```python
from build123d import *

# Parameters (mm, degrees)
F0_W     = 9
F0_H     = 6.4
F0_H_2   = 1.8
F1_DEPTH = 10
F3_DEPTH = 68.4572498646


with BuildPart() as f1:
    # F0 (on Top) → F1 (new body)
    with BuildSketch(Plane.XY):
        with BuildLine():
            Line((-23, -13.2790561914), (-23, -19.4471))
            Line((-23, -19.4471), (-23, -19.4592028655))
            ThreePointArc((-23, -19.4592028655), (-15.9535433508, -25.5567022661), (-7.3808786516, -29.2093))
            Line((-7.3808786516, -29.2093), (0, -29.2093))
            Line((0, -29.2093), (0, 0))
            Line((0, 0), (-11.5, -19.918584287))
            Line((-11.5, -19.918584287), (-23, -13.2790561914))
        make_face()
        with BuildLine():
            Line((-23, -19.4592028655), (-23, -19.4471))
            Line((-23, -19.4471), (-23, -13.2790561914))
            Line((-23, -13.2790561914), (-28.3416826299, -10.195034287))
            Line((-28.3416826299, -10.195034287), (-28.3521640189, -10.1889828543))
            ThreePointArc((-28.3521640189, -10.1889828543), (-26.0910987143, -15.0637028662), (-23, -19.4592028655))
        make_face()
        with BuildLine():
            ThreePointArc((-7.3808786516, -29.2093), (-15.9535433508, -25.5567022661), (-23, -19.4592028655))
            Line((-23, -19.4592028655), (-23, -31.0093))
            Line((-23, -31.0093), (-14, -31.0093))
            Line((-14, -31.0093), (-14, -29.2093))
            Line((-14, -29.2093), (-7.3808786516, -29.2093))
        make_face()
        with BuildLine():
            Line((-28.3416826299, -10.195034287), (-23, -13.2790561914))
            Line((-23, -13.2790561914), (-23, 0))
            Line((-23, 0), (0, 0))
            Line((0, 0), (-25.2959958268, 14.60465))
            Line((-25.2959958268, 14.60465), (-28.9864351526, 8.2126215854))
            ThreePointArc((-28.9864351526, 8.2126215854), (-30.1095250747, -1.0378226891), (-28.3521640189, -10.1889828543))
            Line((-28.3521640189, -10.1889828543), (-28.3416826299, -10.195034287))
        make_face()
        Polygon((-23, 0), (-23, -13.2790561914), (-11.5, -19.918584287), (0, 0), align=None)
        with Locations((-18.5, -34.2093)):
            Rectangle(F0_W, F0_H)
        with BuildLine():
            Line((-38.3548415536, -4.413934287), (-28.3521640189, -10.1889828543))
            ThreePointArc((-28.3521640189, -10.1889828543), (-30.1095250747, -1.0378226891), (-28.9864351526, 8.2126215854))
            Line((-28.9864351526, 8.2126215854), (-32.2959958268, 2.480294347))
            Line((-32.2959958268, 2.480294347), (-33.8548415536, 3.380294347))
            Line((-33.8548415536, 3.380294347), (-38.3548415536, -4.413934287))
        make_face()
        with Locations((-18.5, -38.3093)):
            Rectangle(F0_W, F0_H_2)
        Polygon((-43.8974041378, -1.213934287), (-38.3548415536, -4.413934287), (-33.8548415536, 3.380294347), (-39.3974041378, 6.580294347), align=None)
        with BuildLine():
            Line((0, 0), (0, -29.2093))
            Line((0, -29.2093), (7.3808786516, -29.2093))
            ThreePointArc((7.3808786516, -29.2093), (15.9535433508, -25.5567022661), (23, -19.4592028655))
            Line((23, -19.4592028655), (23, -19.4471))
            Line((23, -19.4471), (23, -13.2790561914))
            Line((23, -13.2790561914), (11.5, -19.918584287))
            Line((11.5, -19.918584287), (0, 0))
        make_face()
        with BuildLine():
            Line((25.2959958268, 14.60465), (0, 0))
            Line((0, 0), (23, 0))
            Line((23, 0), (23, -13.2790561914))
            Line((23, -13.2790561914), (28.3416826299, -10.195034287))
            Line((28.3416826299, -10.195034287), (28.3521640189, -10.1889828543))
            ThreePointArc((28.3521640189, -10.1889828543), (29.6802773315, -5.1712390862), (30.1274057323, 0))
            ThreePointArc((30.1274057323, 0), (29.8407998279, 4.1457498468), (28.9864351526, 8.2126215854))
            Line((28.9864351526, 8.2126215854), (25.2959958268, 14.60465))
        make_face()
        with BuildLine():
            Line((11.5, 19.918584287), (0, 0))
            Line((0, 0), (25.2959958268, 14.60465))
            Line((25.2959958268, 14.60465), (21.6055565009, 20.9966784146))
            ThreePointArc((21.6055565009, 20.9966784146), (14.155981724, 26.5945249552), (5.3521640189, 29.6481857198))
            Line((5.3521640189, 29.6481857198), (5.3416826299, 29.642134287))
            Line((5.3416826299, 29.642134287), (0, 26.5581123827))
            Line((0, 26.5581123827), (11.5, 19.918584287))
        make_face()
        with BuildLine():
            Line((-25.2959958268, 14.60465), (0, 0))
            Line((0, 0), (-11.5, 19.918584287))
            Line((-11.5, 19.918584287), (0, 26.5581123827))
            Line((0, 26.5581123827), (-5.3416826299, 29.642134287))
            Line((-5.3416826299, 29.642134287), (-5.3521640189, 29.6481857198))
            ThreePointArc((-5.3521640189, 29.6481857198), (-14.155981724, 26.5945249552), (-21.6055565009, 20.9966784146))
            Line((-21.6055565009, 20.9966784146), (-25.2959958268, 14.60465))
        make_face()
        Polygon((23, 0), (0, 0), (11.5, -19.918584287), (23, -13.2790561914), align=None)
        Polygon((-11.5, 19.918584287), (0, 0), (11.5, 19.918584287), (0, 26.5581123827), align=None)
        Polygon((-45.4562498646, -0.313934287), (-43.8974041378, -1.213934287), (-39.3974041378, 6.580294347), (-40.9562498646, 7.480294347), align=None)
        with BuildLine():
            ThreePointArc((23, -19.4592028655), (15.9535433508, -25.5567022661), (7.3808786516, -29.2093))
            Line((7.3808786516, -29.2093), (14, -29.2093))
            Line((14, -29.2093), (14, -31.0093))
            Line((14, -31.0093), (23, -31.0093))
            Line((23, -31.0093), (23, -19.4592028655))
        make_face()
        with Locations((18.5, -34.2093)):
            Rectangle(F0_W, F0_H)
        with BuildLine():
            Line((-18.2959958268, 26.729005653), (-21.6055565009, 20.9966784146))
            ThreePointArc((-21.6055565009, 20.9966784146), (-14.155981724, 26.5945249552), (-5.3521640189, 29.6481857198))
            Line((-5.3521640189, 29.6481857198), (-15.3548415536, 35.423234287))
            Line((-15.3548415536, 35.423234287), (-19.8548415536, 27.629005653))
            Line((-19.8548415536, 27.629005653), (-18.2959958268, 26.729005653))
        make_face()
        with BuildLine():
            Line((23, -19.4471), (23, -19.4592028655))
            ThreePointArc((23, -19.4592028655), (26.0910987143, -15.0637028662), (28.3521640189, -10.1889828543))
            Line((28.3521640189, -10.1889828543), (28.3416826299, -10.195034287))
            Line((28.3416826299, -10.195034287), (23, -13.2790561914))
            Line((23, -13.2790561914), (23, -19.4471))
        make_face()
        with BuildLine():
            ThreePointArc((5.3521640189, 29.6481857198), (14.155981724, 26.5945249552), (21.6055565009, 20.9966784146))
            Line((21.6055565009, 20.9966784146), (18.2959958268, 26.729005653))
            Line((18.2959958268, 26.729005653), (19.8548415536, 27.629005653))
            Line((19.8548415536, 27.629005653), (15.3548415536, 35.423234287))
            Line((15.3548415536, 35.423234287), (5.3521640189, 29.6481857198))
        make_face()
        with BuildLine():
            Line((32.2959958268, 2.480294347), (28.9864351526, 8.2126215854))
            ThreePointArc((28.9864351526, 8.2126215854), (29.8407998279, 4.1457498468), (30.1274057323, 0))
            ThreePointArc((30.1274057323, 0), (29.6802773315, -5.1712390862), (28.3521640189, -10.1889828543))
            Line((28.3521640189, -10.1889828543), (38.3548415536, -4.413934287))
            Line((38.3548415536, -4.413934287), (33.8548415536, 3.380294347))
            Line((33.8548415536, 3.380294347), (32.2959958268, 2.480294347))
        make_face()
        with BuildLine():
            Line((-5.3416826299, 29.642134287), (0, 26.5581123827))
            Line((0, 26.5581123827), (5.3416826299, 29.642134287))
            Line((5.3416826299, 29.642134287), (5.3521640189, 29.6481857198))
            ThreePointArc((5.3521640189, 29.6481857198), (0, 30.1274057323), (-5.3521640189, 29.6481857198))
            Line((-5.3521640189, 29.6481857198), (-5.3416826299, 29.642134287))
        make_face()
        with Locations((18.5, -38.3093)):
            Rectangle(F0_W, F0_H_2)
        Polygon((-25.3974041378, 30.829005653), (-19.8548415536, 27.629005653), (-15.3548415536, 35.423234287), (-20.8974041378, 38.623234287), align=None)
        Polygon((-26.9562498646, 31.729005653), (-25.3974041378, 30.829005653), (-20.8974041378, 38.623234287), (-22.4562498646, 39.523234287), align=None)
        Polygon((33.8548415536, 3.380294347), (38.3548415536, -4.413934287), (43.8974041378, -1.213934287), (39.3974041378, 6.580294347), align=None)
        Polygon((15.3548415536, 35.423234287), (19.8548415536, 27.629005653), (25.3974041378, 30.829005653), (20.8974041378, 38.623234287), align=None)
        Polygon((39.3974041378, 6.580294347), (43.8974041378, -1.213934287), (45.4562498646, -0.313934287), (40.9562498646, 7.480294347), align=None)
        Polygon((20.8974041378, 38.623234287), (25.3974041378, 30.829005653), (26.9562498646, 31.729005653), (22.4562498646, 39.523234287), align=None)
    extrude(amount=-F1_DEPTH)

    # F2 (on face) → F3 (cut, through all)
    with BuildSketch(Plane.YZ.offset(23)):
        with BuildLine():
            ThreePointArc((-33.9093, -1.7), (-37.2093, -5), (-33.9093, -8.3))
            Line((-33.9093, -8.3), (-33.9093, -1.7))
        make_face()
        with BuildLine():
            Line((-33.9093, -1.7), (-33.9093, -8.3))
            ThreePointArc((-33.9093, -8.3), (-31.5758476221, -7.3334523779), (-30.6093, -5))
            ThreePointArc((-30.6093, -5), (-31.5758476221, -2.6665476221), (-33.9093, -1.7))
        make_face()
    extrude(amount=-F3_DEPTH, mode=Mode.SUBTRACT)


solid = f1.part
```
Verification items for the finished model (mm, model axes). A direction names the side the tool comes from. Round coordinates to 2 decimals unless told otherwise and drop trailing zeros. Order: outer loops, then holes, each group sorted by start corner. A loop starts at its lowest first (then second) coordinate and runs counter-clockwise, first axis right, second up. Notation, with made-up numbers: (79, 26) - (111, 26) arc R26 ccw to (111, 54) - close; hole circle Ø5 at (15, 67). An arc over 180 degrees is marked (long way). Use CSV: the item, a comma, the result in double quotes. Start each with the question number.
1) Section check C-C, the plane y = -16. Record the cut outline in (x, z), plus the area to 3 significant figures.
2) Access from +Z, -Z, +X, -X, +Y, -Y to the whole of each face (thin tool, end or side, straight path). Record for faces 1 (the flat face through (43.238, 3.529, -4.93)), 2 (the flat face through (-14, -37, -3)).
3) Section check D-D, the plane x = -11. Record the cut outline in (y, z).
4) Section check B-B, the plane z = -4. State how many separate pieces and enclosed holes the cut face has, plus the area to 3 significant figures.
5) Section check A-A, the plane x = 16.5. Record the cut outline in (y, z).
6) Thickness scan on L1, parallel to Y at x = 20.5, z = -2.75; L2, parallel to Y at x = -22.5, z = -4.25; L3, parallel to X at y = 3.5, z = -7. Record the ranges inside material, lowest first.
7) Mould release check, pull along X, two halves, no side actions. Record for faces 3 (the flat face through (23, -29, -5)), 4 (the flat face through (0, -29.209, -5)), 5 (the flat face through (-23, -29, -5)), 6 (the flat face through (14, -37.5, -4.9)): +X half, -X half, draft (parallel to the pull), parting line (faces both ways), or undercut.
8) Go/stop test with flat-tipped pins: P1, Ø4, axis at x = -22, y = 25.5, coming from the +Z side; P2, Ø1.5, axis at x = 10, z = -8, coming from the -Y side; P3, Ø4, axis at x = -1, y = 8, coming from the +Z side; P4, Ø1.5, axis at x = -14, z = -2, coming from the +Y side. Record where each tip stops, or that it passes through.
Answers:
1,outline,"(-25.53, -10) - (25.53, -10) - (25.53, 0) - (-25.53, 0) - close"
1,area,"511 mm²"
2,face 1,"+Z, -Z, +X, +Y"
2,face 2,"+Z, -Z, -Y"
3,outline,"(-29.21, -10) - (32.91, -10) - (32.91, 0) - (-29.21, 0) - close"
4,separate pieces,"3"
4,enclosed holes,"0"
4,area,"3,600 mm²"
5,outline,"(-39.21, -10) - (36.08, -10) - (36.08, 0) - (-39.21, 0) - close; hole circle Ø6.6 at (-33.91, -5)"
6,L1,"y = -39.21 to -36.32, -31.5 to 22.91, 28 to 38.39"
6,L2,"y = -39.21 to -37.12, -30.7 to 19.45, 29.16 to 39.45"
6,L3,"x = -43.25 to -34.06, -31.71 to 31.71, 34.06 to 43.25"
7,face 3,"+X half"
7,face 4,"undercut"
7,face 5,"-X half"
7,face 6,"undercut"
8,P1,"passes through"
8,P2,"stops at y = -29.21"
8,P3,"stops at z = 0"
8,P4,"stops at y = 35.07"
